```python
from build123d import *

# Parameters (mm, degrees)
SKETCH_1_R            = 2.5
EXTRUDE_1_DEPTH       = 15
CUT_EXTRUDE_START     = -8.5
SKETCH_4_W            = 25.510318362
SKETCH_4_H            = 11.123148158
CUT_EXTRUDE_1_DEPTH   = 10.5
SKETCH_5_R            = 8
CUT_EXTRUDE_2_DEPTH   = 45.795847434
SKETCH_6_R            = 2
CUT_EXTRUDE_3_DEPTH   = 38.665208712
SKETCH_7_W            = 21.685962805
SKETCH_7_H            = 6.466354348
CUT_EXTRUDE_2_2_DEPTH = 45.795847434
SKETCH_8_R            = 2
CUT_EXTRUDE_4_DEPTH   = 37.741229529


with BuildPart() as part:
    # Эскиз1 → Вытянуть1 (new body)
    with BuildSketch(Plane(origin=(0, 0, 0), x_dir=(1, 0, 0), z_dir=(0, 1, 0))):
        Polygon((14, 26.964204166), (7.131727139, 31.585882089), (-7.131727139, 31.585882089), (-14, 26.964204166), (-14, -27.88029884), (14, -27.88029884), align=None)
        with Locations(Location((0, 25.393583102, 0), (0, 0, 270))):
            Circle(SKETCH_1_R, mode=Mode.SUBTRACT)
    extrude(amount=EXTRUDE_1_DEPTH)

    # Эскиз4 → Вырез-Вытянуть1 (cut)
    with BuildSketch(Plane(origin=(14, 0, 0), x_dir=(0, 0, -1), z_dir=(1, 0, 0)).offset(CUT_EXTRUDE_START)):
        with Locations((-6.426786787, 9.438425921)):
            Rectangle(SKETCH_4_W, SKETCH_4_H)
    extrude(amount=-CUT_EXTRUDE_1_DEPTH, mode=Mode.SUBTRACT)

    # Эскиз5 → Cut-Extrude 2 (cut, through all)
    with BuildSketch(Plane(origin=(14, 0, 0), x_dir=(0, 0, -1), z_dir=(1, 0, 0))):
        with Locations((-6.37029618, 15)):
            Circle(SKETCH_5_R)
    extrude(amount=-CUT_EXTRUDE_2_DEPTH, mode=Mode.SUBTRACT)

    # Эскиз6 → Вытянуть3 (cut, through all)
    with BuildSketch(Plane(origin=(0, 15, 0), x_dir=(1, 0, 0), z_dir=(0, 1, 0))):
        with Locations(Location((-9.761047482, -23.411554498, 0), (0, 0, 270))):
            Circle(SKETCH_6_R)
        with Locations(Location((9.761047482, -23.411554498, 0), (0, 0, 90))):
            Circle(SKETCH_6_R)
    extrude(amount=-CUT_EXTRUDE_3_DEPTH, mode=Mode.SUBTRACT)

    # Эскиз7 → Cut-Extrude 2 2 (cut, through all)
    with BuildSketch(Plane.ZY.offset(14)):
        with Locations((-20.742900687, 15.733177174)):
            Rectangle(SKETCH_7_W, SKETCH_7_H)
    extrude(amount=-CUT_EXTRUDE_2_2_DEPTH, mode=Mode.SUBTRACT)

    # Эскиз8 → Вытянуть4 (cut, through all)
    with BuildSketch(Plane(origin=(0, 12.5, 0), x_dir=(1, 0, 0), z_dir=(0, 1, 0))):
        with Locations(Location((-10.080038917, 12.621065786, 0), (0, 0, 270))):
            Circle(SKETCH_8_R)
        with Locations(Location((10.080038917, 12.621065786, 0), (0, 0, 270))):
            Circle(SKETCH_8_R)
    extrude(amount=-CUT_EXTRUDE_4_DEPTH, mode=Mode.SUBTRACT)


solid = part.part
```
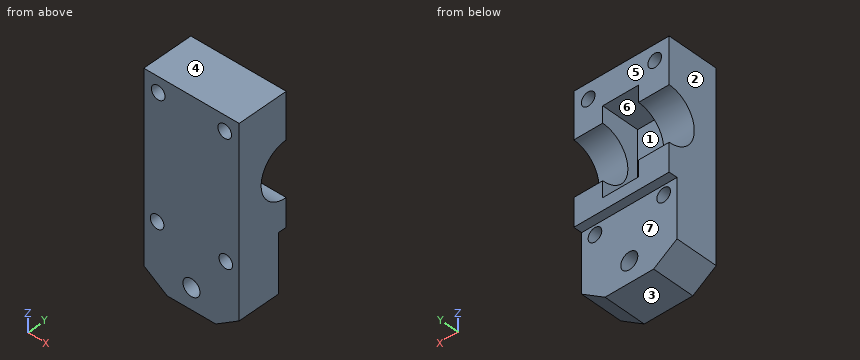
Read the model definition and answer for the solid it produces. Units are mm, in the model's axes. Face numbers are marked on the shaded views. A direction names the side the tool comes from. Coordinates: 2 decimals unless noted, no trailing zeros. Write each loop counter-clockwise with the first axis right and the second up, starting at its lowest first coordinate (ties: lowest second). Pieces come first, ordered by that corner, then holes. Notation, with made-up numbers: (76.25, 72) -> (114.25, 72) arc R19 ccw to (114.25, 103) -> close; hole circle Ø2 at (-10, -18). An arc over 180 degrees is marked (long way). Return JSON: item names as keys, results as strings.
1. Determine the mould class of the marked faces 1, 2, 3 and 4 for opening direction Z: pulls with the +Z half, pulls with the -Z half, needs draft (parallel to the pull), parting line crosses it, or undercut.
Found:
{"face 1": "undercut", "face 2": "needs draft", "face 3": "pulls with the -Z half", "face 4": "pulls with the +Z half"}
2. A cutting plane is placed at B-B (x = 0). Determine the outline of the cut face in (y, z), and give its area (3 significant figures).
Found:
{"outline": "(0, -31.59) -> (12.5, -31.59) -> (12.5, -27.89) -> (0, -27.89) -> close; (0, -22.89) -> (12.5, -22.89) -> (12.5, -9.9) -> (15, -9.9) -> (15, -6.33) -> (3.88, -6.33) -> (3.88, 19.18) -> (15, 19.18) -> (15, 27.88) -> (0, 27.88) -> close", "area": "492 mm2"}
3. A cutting plane is placed at C-C (z = 16). Determine the outline of the cut face in (x, y), and give its area (3 significant figures).
Found:
{"outline": "(-14, 0) -> (14, 0) -> (14, 15) -> (5.5, 15) -> (5.5, 3.88) -> (-5, 3.88) -> (-5, 15) -> (-14, 15) -> close", "area": "303 mm2"}
4. A cutting plane is placed at A-A (y = 14.25). Determine the outline of the cut face in (x, z).
Found:
{"outline": "(-14, -9.9) -> (14, -9.9) -> (14, -1.59) -> (5.5, -1.59) -> (5.5, -6.33) -> (-5, -6.33) -> (-5, -1.59) -> (-14, -1.59) -> close; (-14, 14.34) -> (-5, 14.34) -> (-5, 19.18) -> (5.5, 19.18) -> (5.5, 14.34) -> (14, 14.34) -> (14, 27.88) -> (-14, 27.88) -> close; hole circle Ø4 at (-9.76, 23.41); hole circle Ø4 at (9.76, 23.41)"}
5. A tool of negligible diameter and unlimited length cuts with its end or side. For the marked faces 5, 6 and 7, from which of +Z, -Z, +X, -X, +Y, -Y can it reach the whole face along a straight path? Write none if from no direction.
Found:
{"face 5": "+Z, -Z, +X, -X, +Y", "face 6": "+Y", "face 7": "-Z, +X, -X, +Y"}
6. A cutting plane is placed at D-D (z = -11.5). Determine the outline of the cut face in (x, y), and give its area (3 significant figures).
Found:
{"outline": "(-14, 0) -> (-11.74, 0) -> (-11.74, 12.5) -> (-14, 12.5) -> close; (-8.42, 0) -> (8.42, 0) -> (8.42, 12.5) -> (-8.42, 12.5) -> close; (11.74, 0) -> (14, 0) -> (14, 12.5) -> (11.74, 12.5) -> close", "area": "267 mm2"}
7. Each of these flat-tipped pins is pushed along its axis until it touches: P1, Ø2, axis at x = -4, y = 14, coming from the -Z side; P2, Ø6, axis at y = 11.5, z = 3, coming from the -X side; P3, Ø3, axis at x = 1.5, z = 12, coming from the +Y side. Where does it stop, or does it pass through?
Found:
{"P1": "z = -9.9", "P2": "through", "P3": "y = 3.88"}
8. Find the intervals of material crossed by line 1 along Z through (x, y) = (0, 7.5); line 2 along X through (y, z) = (7.5, -4); line 3 along Z through (x, y) = (-3.5, 8.25), in increasing order. Write a range as from..to.
Found:
{"line 1": "-31.59..-27.89, -22.89..-6.33, 19.18..27.88", "line 2": "-14..-5, 5.5..14", "line 3": "-31.59..-6.33, 19.18..27.88"}
